Verification items for the finished model (mm, model axes). A direction names the side the tool comes from. Round coordinates to 2 decimals unless told otherwise and drop trailing zeros. Write each loop counter-clockwise with the first axis right and the second up, starting at its lowest first coordinate (ties: lowest second). Pieces come first, ordered by that corner, then holes. Notation, with made-up numbers: M 42.5,-32.5 L 75.5,-32.5 A33 ccw 75.5,-1.5 Z; hole C 6,11.5 d3. An arc over 180 degrees is marked long. Write each question's results on one line, items separated by ' | '.
from build123d import *

# Parameters (mm, degrees)
SKETCH1_W           = 25.4
SKETCH1_H           = 6.35
BOSS_EXTRUDE1_DEPTH = 100
SKETCH2_R           = 2.1
CUT_EXTRUDE1_DEPTH  = 110.906322202
SKETCH2_3_R         = 5
CUT_EXTRUDE2_DEPTH  = 4
SKETCH2_4_R         = 5
CUT_EXTRUDE3_DEPTH  = 4
SKETCH5_W           = 25.4
SKETCH5_H           = 5
SKETCH5_H_2         = 12
CUT_EXTRUDE4_DEPTH  = 110.906322202
SKETCH6_R           = 5.25
CUT_EXTRUDE5_DEPTH  = 106.377415322
SKETCH7_W           = 25.4
SKETCH7_H           = 3.7
CUT_EXTRUDE6_DEPTH  = 106.377415322
BOSS_EXTRUDE2_START = -2.35
SKETCH8_R           = 5.25
SKETCH8_R_2         = 3
BOSS_EXTRUDE2_DEPTH = 2.35


with BuildPart() as part:
    # Sketch1 → Boss-Extrude1 (new body)
    with BuildSketch(Plane(origin=(0, 0, 0), x_dir=(1, 0, 0), z_dir=(0, 1, 0))):
        with Locations((32.456141995, 0.058688594)):
            Rectangle(SKETCH1_W, SKETCH1_H)
    extrude(amount=BOSS_EXTRUDE1_DEPTH)

    # Sketch2 → Cut-Extrude1 (cut, through all)
    with BuildSketch(Plane.XY.offset(3.116311406)):
        with Locations((32.456141995, 81.7)):
            Circle(SKETCH2_R)
        with Locations((32.456141995, 23.71)):
            Circle(SKETCH2_R)
    extrude(amount=-CUT_EXTRUDE1_DEPTH, mode=Mode.SUBTRACT)

    # Sketch2_3 → Cut-Extrude2 (cut)
    with BuildSketch(Plane.XY.offset(3.116311406)):
        with Locations((32.456141995, 81.7)):
            Circle(SKETCH2_3_R)
    extrude(amount=-CUT_EXTRUDE2_DEPTH, mode=Mode.SUBTRACT)

    # Sketch2_4 → Cut-Extrude3 (cut)
    with BuildSketch(Plane.XY.offset(3.116311406)):
        with Locations((32.456141995, 23.71)):
            Circle(SKETCH2_4_R)
    extrude(amount=-CUT_EXTRUDE3_DEPTH, mode=Mode.SUBTRACT)

    # Sketch5 → Cut-Extrude4 (cut, through all)
    with BuildSketch(Plane.XY.offset(3.116311406)):
        with Locations((32.456141995, 97.5)):
            Rectangle(SKETCH5_W, SKETCH5_H)
        with Locations((32.456141995, 6)):
            Rectangle(SKETCH5_W, SKETCH5_H_2)
    extrude(amount=-CUT_EXTRUDE4_DEPTH, mode=Mode.SUBTRACT)

    # Sketch6 → Cut-Extrude5 (cut, through all)
    with BuildSketch(Plane.XY.offset(3.116311406)):
        with Locations((32.456141995, 53.471)):
            Circle(SKETCH6_R)
    extrude(amount=-CUT_EXTRUDE5_DEPTH, mode=Mode.SUBTRACT)

    # Sketch7 → Cut-Extrude6 (cut, through all)
    with BuildSketch(Plane.XY.offset(3.116311406)):
        with Locations((32.456141995, 13.85)):
            Rectangle(SKETCH7_W, SKETCH7_H)
    extrude(amount=-CUT_EXTRUDE6_DEPTH, mode=Mode.SUBTRACT)

    # Sketch8 → Boss-Extrude2 (add)
    with BuildSketch(Plane(origin=(0, 0, -3.233688594), x_dir=(-1, 0, 0), z_dir=(0, 0, -1)).offset(BOSS_EXTRUDE2_START)):
        with Locations(Location((-32.456141995, 53.471, 0), (0, 0, 180))):
            Circle(SKETCH8_R)
        with Locations((-32.456141995, 53.471)):
            Circle(SKETCH8_R_2, mode=Mode.SUBTRACT)
    extrude(amount=BOSS_EXTRUDE2_DEPTH)


solid = part.part
1) Material ranges on line 1 (Y direction, x = 36.25, z = 2); line 2 (Y direction, x = 34.25, z = 1); line 3 (Z direction, x = 28.75, y = 83), recorded low to high. Write a range as [from, to].
Calculated:
line 1: y = [15.7, 20.45], [26.97, 49.84], [57.1, 78.44], [84.96, 95] | line 2: y = [15.7, 19.04], [28.38, 48.54], [58.41, 77.03], [86.37, 95] | line 3: z = [-3.23, -0.88]
2) Depth check by flat-ended pin: P1, Ø5.5, axis at x = 32.46, y = 81.7, coming from the +Z side. Enter the tip coordinate at first touch or a pass-through.
Calculated:
P1: stops at z = -0.88
3) Draft check along X on faces 3 (the flat face through (19.756, 55, 0)), 4 (the flat face through (45.156, 55, 0)), 5 (the flat face through (35, 56, -0.884)), 6 (the flat face through (32, 95, 0)). Enter one of: pulls with the +X half, pulls with the -X half, needs draft (parallel to the pull), parting line crosses it, or undercut.
Calculated:
face 3: pulls with the -X half | face 4: pulls with the +X half | face 5: undercut | face 6: needs draft
4) Sectioned sample at C-C, the plane y = 81. Record the cut outline in (x, z).
Calculated:
outline: M 19.76,-3.23 L 30.48,-3.23 L 30.48,-0.88 L 27.51,-0.88 L 27.51,3.12 L 19.76,3.12 Z; M 34.44,-3.23 L 45.16,-3.23 L 45.16,3.12 L 37.41,3.12 L 37.41,-0.88 L 34.44,-0.88 Z
5) Sectioned sample at B-B, the plane z = -2. Record the cut outline in (x, y), and give its area (3 significant figures).
Calculated:
outline: M 19.76,15.7 L 45.16,15.7 L 45.16,95 L 19.76,95 Z; hole C 32.46,53.47 d6; hole C 32.46,23.71 d4.2; hole C 32.46,81.7 d4.2 | area: 1,960 mm²
6) Sectioned sample at A-A, the plane y = 23.71. Record the cut outline in (x, z), and give its area (3 significant figures).
Calculated:
outline: M 19.76,-3.23 L 30.36,-3.23 L 30.36,-0.88 L 27.46,-0.88 L 27.46,3.12 L 19.76,3.12 Z; M 34.56,-3.23 L 45.16,-3.23 L 45.16,3.12 L 37.46,3.12 L 37.46,-0.88 L 34.56,-0.88 Z | area: 111 mm²
7) Access from +Z, -Z, +X, -X, +Y, -Y to the whole of each face (thin tool, end or side, straight path). Record for faces 1 (the flat face through (29, 55, -3.234)), 2 (the cylindrical face through (31.37, 76.82, 1.14)).
Calculated:
face 1: -Z, +X, -X, +Y, -Y | face 2: +Z
